Check sheet for the drawn part. Datum: minimum x, y, z corner. Units: mm. Round coordinates to 2 decimals unless told otherwise and drop trailing zeros. Write each loop counter-clockwise with the first axis right and the second up, starting at its lowest first coordinate (ties: lowest second). Pieces come first, ordered by that corner, then holes. Notation, with made-up numbers: M 33.25,-8 L 50.25,-8 A33 ccw 50.25,27 Z; hole C 80.5,-1.5 d8. An arc over 180 degrees is marked long. One line per item, written item: value. Start each with the question number.
1. Scan lines: probe 1 along Z at (x, y) = (43, 1.75); probe 2 along X at (y, z) = (0.65, 7) (1 decimal); probe 3 along X at (y, z) = (0.9, 19.5) (1 decimal). Record each from-to range of solid material in increasing order. Write a range as [from, to].
2. Section check B-B (z = 20.5). Record the boundary of the cut face in (x, y), and give its area (3 significant figures).
3. Section check D-D (x = 24). Record the boundary of the cut face in (y, z).
4. Depth check by flat-ended pin: P1, Ø10, axis at x = 43.5, z = 5, coming from the +Y side; P2, Ø1, axis at x = 27.5, y = 1, coming from the +Z side; P3, Ø1, axis at x = 35.5, y = 1, coming from the +Z side. Enter the tip coordinate at first touch or a pass-through.
5. Section check A-A (y = 2.5). Record the boundary of the cut face in (x, z), and give its area (3 significant figures).
6. Section check C-C (x = 52). Record the boundary of the cut face in (y, z), and give its area (3 significant figures).
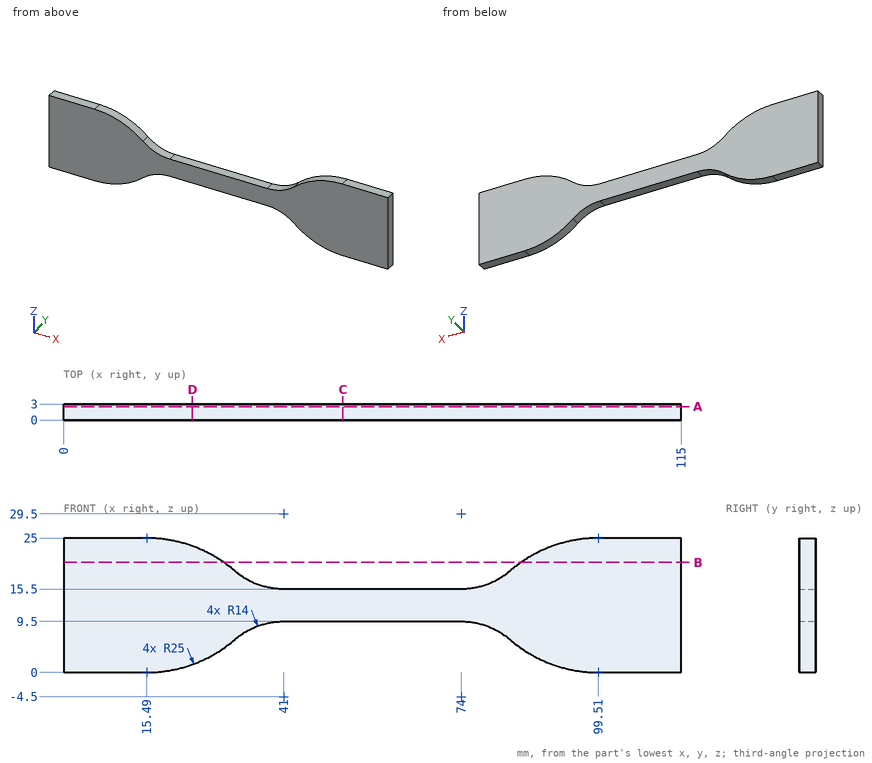
Result sheet:
1. probe 1: z = [9.5, 15.5]
1. probe 2: x = [0, 33], [82, 115]
1. probe 3: x = [0, 31.1], [83.9, 115]
2. outline: M 0,0 L 29.8,0 L 29.8,3 L 0,3 Z; M 85.2,0 L 115,0 L 115,3 L 85.2,3 Z
2. area: 179 mm2
3. outline: M 0,1.49 L 3,1.49 L 3,23.51 L 0,23.51 Z
4. P1: stops at y = 3
4. P2: stops at z = 22.19
4. P3: stops at z = 16.85
5. outline: M 0,0 L 15.49,0 A25 ccw 31.84,6.09 A14 cw 41,9.5 L 74,9.5 A14 cw 83.16,6.09 A25 ccw 99.51,0 L 115,0 L 115,25 L 99.51,25 A25 ccw 83.16,18.91 A14 cw 74,15.5 L 41,15.5 A14 cw 31.84,18.91 A25 ccw 15.49,25 L 0,25 Z
5. area: 1,810 mm2
6. outline: M 0,9.5 L 3,9.5 L 3,15.5 L 0,15.5 Z
6. area: 18.0 mm2
